Autodesk Inventor part; units mm, degrees
ref_plane "YZ Plane" through (0, 0, 0) normal (1, 0, 0) x (0, 1, 0)
ref_plane "XZ Plane" through (0, 0, 0) normal (0, 1, 0) x (-1, 0, 0)
ref_plane "XY Plane" through (0, 0, 0) normal (0, 0, 1) x (1, 0, 0)
sketch "Sketch1" plane through (0, 0, 0) normal (0, 1, 0) x (-1, 0, 0)
  circle A0 centre (0, 0) radius 13.5
  line L0 (0, -13.5) -> (30, -13.5) construction
  line L1 (0, 13.5) -> (30, 13.5) construction
  line L2 (30, 13.5) -> (30, -13.5) construction
  line L3 (0, -13.5) -> (16, -13.5) construction
  line L4 (0, 13.5) -> (16, 13.5) construction
  line L5 (16, 13.5) -> (16, -13.5) construction
  line L6 (30, 13.5) -> (30, 9.5) construction
  line L7 (30, -13.5) -> (30, -9.5) construction
  line L8 (0, -13.5) -> (0, -16.5) construction
  line L9 (0, 13.5) -> (0, 16.5) construction
  line L10 (30, -2.5) -> (33, -2.5) construction
  line L11 (-13.5, 0) -> (-16.5, 0) construction
  line L12 (33, -2.5) -> (33, -16.5)
  line L13 (33, -16.5) -> (0, -16.5)
  line L14 (33, -2.5) -> (33, 16.5)
  line L15 (33, 16.5) -> (0, 16.5)
  line L16 (0, 16.5) -> (-16.5, 16.5)
  line L17 (-16.5, 0) -> (-16.5, 16.5)
  line L18 (0, -16.5) -> (-16.5, -16.5)
  line L19 (-16.5, -16.5) -> (-16.5, 0)
  line L20 (0, 13.5) -> (14, 13.5) construction
  line L21 (0, -13.5) -> (14, -13.5) construction
  line L22 (14, 13.5) -> (14, -13.5) construction
  line L23 (33, 9.5) -> (33, 10.5) construction
  line L24 (33, -9.5) -> (33, -10.5) construction
  line L25 (14, -11.5) -> (14, -6.5) construction
  line L26 (14, 10.5) -> (14, 5.5) construction
  line L27 (0, -13.5) -> (15, -13.5) construction
  line L28 (0, 13.5) -> (15, 13.5) construction
  line L29 (15, 13.5) -> (15, -13.5) construction
  line L30 (14, -11.5) -> (14, -6.5) construction
  line L31 (14, -13.5) -> (14, -8.5) construction
  line L32 (14, 13.5) -> (14, 8.5) construction
  line L33 (14, 8.5) -> (30, 8.5) construction
  line L34 (14, -8.5) -> (30, -8.5) construction
  line L35 (16, -8.5) -> (16, -9.5) construction
  line L36 (16, 8.5) -> (16, 9.5) construction
  line L37 (16, 8.5) -> (16, 7.5) construction
  line L38 (16, -8.5) -> (16, -7.5) construction
  line L39 (30, -9.5) -> (14, -9.5) construction
  line L40 (30, 9.5) -> (14, 9.5) construction
  line L41 (14, -9.5) -> (33, -9.5)
  line L42 (14, 9.5) -> (33, 9.5)
  line L43 (33, 8.5) -> (15, 8.5)
  line L44 (15, 8.5) -> (15, -8.5)
  line L45 (15, -8.5) -> (33, -8.5)
  line L46 (14, -9.5) -> (14, 9.5)
  line L47 (33, -9.5) -> (33, 8.5)
  dimension "d0" = 27
  dimension "d1" = 30
  dimension "d2" = 30
  dimension "d3" = 16
  dimension "d4" = 16
  dimension "d5" = 4
  dimension "d6" = 4
  dimension "d7" = 3
  dimension "d8" = 3
  dimension "d9" = 3
  dimension "d10" = 3
  dimension "d16" = 14
  dimension "d17" = 14
  dimension "d26" = 15
  dimension "d27" = 15
  dimension "d29" = 5
  dimension "d30" = 5
  dimension "d31" = 1
  dimension "d32" = 1
  dimension "d33" = 1
  dimension "d34" = 1
extrude "Extrusion5" add sketch "Sketch1" against normal blind 2.5 contours L12 L13 L18 L19 L17 L16 L15 L14 L42 L46 L41
extrude "Extrusion6" add sketch "Sketch1" against normal blind 10 contours L12 L41 L46 L42 L14 L43 L44 L45
extrude "Extrusion7" add sketch "Sketch1" against normal blind 4 contours L12 L45 L44 L43 L14
properties part number "joystick_test_v2_3DPrint"
CAD build for the part. Positions are in the model's coordinates, mm. A direction names the side the tool comes from. Coordinates: 2 decimals unless noted, no trailing zeros. Order: outer loops, then holes, each group sorted by start corner. A loop starts at its lowest first (then second) coordinate and runs counter-clockwise, first axis right, second up.
Item 1: Pin check, flat tips, straight feed: pin 1 Ø2 at (x, y) = (-22, -5) entering from +Z; pin 2 Ø4 at (y, z) = (-6, 1.5) entering from +X; pin 3 Ø1.5 at (x, z) = (9, 12) entering from -Y; pin 4 Ø1 at (x, z) = (-15.5, -9.5) entering from +Y. Stop position of each tip, or through.
Check sheet entries:
pin 1: stops at z = 9.5
pin 2: stops at x = -14
pin 3: stops at y = -2.5
pin 4: stops at y = 0
Item 2: Two-plate mould, pull along X, no slides. Class faces 5 (the face through (-14, -6, 0)), 6 (the face through (-24, -4, 0)), 7 (the face through (2.93, -1.23, -13.18)): +X half, -X half, draft (parallel to the pull), parting line (faces both ways), or undercut.
Check sheet entries:
face 5: +X half
face 6: draft
face 7: undercut
Item 3: Band-saw the part on D-D on y = -7.5. List the corners of the cut face in (x, z), plus the area to 3 significant figures.
Check sheet entries:
outline: (-33, -9.5) - (-14, -9.5) - (-14, 9.5) - (-33, 9.5) - (-33, 8.5) - (-15, 8.5) - (-15, -8.5) - (-33, -8.5) - close
area: 55.0 mm2
Item 4: Band-saw the part on C-C on x = 0. List the corners of the cut face in (y, z), plus the area to 3 significant figures.
Check sheet entries:
outline: (-2.5, -16.5) - (0, -16.5) - (0, -13.5) - (-2.5, -13.5) - close; (-2.5, 13.5) - (0, 13.5) - (0, 16.5) - (-2.5, 16.5) - close
area: 15.0 mm2
Item 5: 3-axis set-ups, long thin cutter, end or side, ignore diameter. For faces 1 (the face through (-13.4, 0, 3.9)), 2 (the face through (-15, -7, 0)), 3 (the face through (-23, -6, 9.5)), 4 (the face through (-23, -6, -9.5)): which of +Z, -Z, +X, -X, +Y, -Y reach the whole face in a straight line?
Check sheet entries:
face 1: +Z, -Z, +X, -X, +Y
face 2: -X, -Y
face 3: +Z, +X, -X, -Y
face 4: -Z, +X, -X, -Y
Item 6: Drill centre lines: L1, parallel to Z at x = 0, y = -0.8; L2, parallel to Z at x = -19, y = -7.75; L3, parallel to X at y = -0.5, z = 0.5. Where is each one in solid material? Low to high.
Check sheet entries:
L1: z = -16.5 to -13.5, 13.5 to 16.5
L2: z = -9.5 to -8.5, 8.5 to 9.5
L3: x = -33 to -13.49, 13.49 to 16.5
Item 7: Band-saw the part on B-B on x = -30. List the corners of the cut face in (y, z).
Check sheet entries:
outline: (-10, -9.5) - (-2.5, -9.5) - (-2.5, -16.5) - (0, -16.5) - (0, 16.5) - (-2.5, 16.5) - (-2.5, 9.5) - (-10, 9.5) - (-10, 8.5) - (-4, 8.5) - (-4, -8.5) - (-10, -8.5) - close
Item 8: Band-saw the part on A-A on z = 0. List the corners of the cut face in (x, y), plus the area to 4 significant figures.
Check sheet entries:
outline: (-33, -4) - (-15, -4) - (-15, -10) - (-14, -10) - (-14, -2.5) - (-13.5, -2.5) - (-13.5, 0) - (-33, 0) - close; (13.5, -2.5) - (16.5, -2.5) - (16.5, 0) - (13.5, 0) - close
area: 90.75 mm2
